```python
from build123d import *

# Parameters (mm, degrees)
BOSS_EXTRUDE1_DEPTH = 5
SKETCH2_R           = 2
CUT_EXTRUDE1_DEPTH  = 10
FILLET1_R           = 10


with BuildPart() as part:
    # Sketch1 → Boss-Extrude1 (new body)
    with BuildSketch(Plane(origin=(-134.331980559, -86.262659899, 84.991923549), x_dir=(0.395424411, 0.253925843, 0.882701083), z_dir=(-0.742744505, -0.476961006, 0.469934888))):
        Polygon((-449.960059364, 72.073536166), (-410.158714417, 68.091961048), (-418.320943409, -13.500796093), (-458.122288356, -9.519220975), align=None)
        Polygon((-431.102989517, -0.46855114), (-420.804391512, -1.498783702), (-414.832028835, 58.203233718), (-445.379561081, 61.259092621), (-451.351923758, 1.557075201), (-441.053325753, 0.526842639), (-441.351943887, -2.458258232), (-431.40160765, -3.453652011), align=None, mode=Mode.SUBTRACT)
    extrude(amount=BOSS_EXTRUDE1_DEPTH)

    # Sketch2 → Cut-Extrude1 (cut)
    with BuildSketch(Plane(origin=(-138.045703084, -88.647464931, 87.341597987), x_dir=(0.395424411, 0.253925843, 0.882701083), z_dir=(-0.742744505, -0.476961006, 0.469934888))):
        with Locations((-444.834579578, -2.61236419)):
            Circle(SKETCH2_R)
        with Locations((-428.018511338, -4.294579677)):
            Circle(SKETCH2_R)
        with Locations((-438.165441255, 64.054888596)):
            Circle(SKETCH2_R)
        with Locations((-421.349373015, 62.372673109)):
            Circle(SKETCH2_R)
    extrude(amount=-CUT_EXTRUDE1_DEPTH, mode=Mode.SUBTRACT)

    # Fillet1
    fillet1_edges = [part.edges().sort_by_distance(p)[0] for p in [
        (-353.05843578, -141.065625808, -311.013470799),
        (-335.168597716, -134.309312615, -275.880780522),
        (-294.308099004, -205.037739583, -283.08558889),
        (-312.197937067, -211.794052776, -318.218279167),
    ]]
    fillet(fillet1_edges, radius=FILLET1_R)


solid = part.part
```
Part model, mm, in its own coordinate system. A direction names the side the tool comes from. Coordinates: 2 decimals unless noted, no trailing zeros. Write each loop counter-clockwise with the first axis right and the second up, starting at its lowest first coordinate (ties: lowest second). Pieces come first, ordered by that corner, then holes.
Item 1: Which spindle directions (+Z, -Z, +X, -X, +Y, -Y) get a long thin tool onto all of the face, cutting with end or side? Do faces 4 (the face through (-312.45, -208.74, -315.43)), 5 (the face through (-313.198, -199.876, -307.777)). Say none if no direction does.
Item 2: Pin check, flat tips, straight feed: pin 1 (8 mm diameter, centred on x = -319.5, z = -314, fed in from -Y); pin 2 (12 mm diameter, centred on x = -335, z = -285, fed in from +Y); pin 3 (5 mm diameter, centred on y = -182.5, z = -287, fed in from +X); pin 4 (3 mm diameter, centred on x = -309.5, z = -296, fed in from -Y). Stop position of each tip, or through.
Item 3: Probe line 1 (Y direction, x = -302.5, z = -292.5); line 2 (X direction, y = -181, z = -314); line 3 (Z direction, x = -329, y = -152). List the from-to ranges inside material, lowest first.
Item 4: Mould opens along X. For faces 1 (the face through (-331.68, -177.95, -309.34)), 2 (the face through (-314.93, -169.28, -279.46)), 3 (the face through (-337.367, -142.413, -287.506)) say: released by +X, released by -X, zero draft, split by the parting line, or undercut.
Item 5: Slice it at B-B (y = -185.5). Write the cut outline in (x, z), and give its area (3 significant figures).
Item 6: Slice it at A-A (x = -326.5). Write the cut outline in (y, z), and give its area (3 significant figures).
Results found:
1. face 4: -Z, -Y
1. face 5: +Z, +Y
2. pin 1: stops at y = -208.68
2. pin 2: stops at y = -134.64
2. pin 3: stops at x = -305.64
2. pin 4: stops at y = -202.11
3. line 1: y = -206.8 to -201.45, -196.99 to -196.32
3. line 2: x = -332.11 to -325.94
3. line 3: z = -279.79 to -278.77
4. face 1: released by -X
4. face 2: released by +X
4. face 3: undercut
5. outline: (-329.93, -314.24) - (-324.84, -316.84) - (-321.77, -311.98) - (-326.86, -309.39) - close; (-310.14, -282.96) - (-305.05, -285.55) - (-303.05, -282.39) - (-308.14, -279.8) - close
5. area: 53.9 mm2
6. outline: (-191.44, -314.85) - (-182.63, -316.54) - (-177.32, -311.15) - (-186.13, -309.46) - close; (-157.18, -280.07) - (-148.36, -281.77) - (-144.91, -278.26) - (-153.72, -276.56) - close
6. area: 93.3 mm2
